```python
from build123d import *

# Parameters (mm, degrees)
CROQUIS1_W              = 53
CROQUIS1_H              = 24
CROQUIS1_R              = 8.15
CROQUIS1_W_2            = 10.3
CROQUIS1_H_2            = 4
CROQUIS1_W_3            = 9
CROQUIS1_H_3            = 2.5
SALIENTE_EXTRUIR1_DEPTH = 2
CROQUIS2_W              = 53
CROQUIS2_H              = 2
SALIENTE_EXTRUIR2_DEPTH = 16
SALIENTE_EXTRUIR3_DEPTH = 2
SALIENTE_EXTRUIR5_START = -53
SALIENTE_EXTRUIR5_DEPTH = 2
CROQUIS5_R              = 1.65
CROQUIS5_R_2            = 2
CORTAR_EXTRUIR1_DEPTH   = 2
REDONDEO1_R             = 2
REDONDEO6_R             = 1


with BuildPart() as part:
    # Croquis1 → Saliente-Extruir1 (new body)
    with BuildSketch(Plane.XY):
        with Locations((26.5, 12)):
            Rectangle(CROQUIS1_W, CROQUIS1_H)
        with Locations((13.5, 12)):
            Circle(CROQUIS1_R, mode=Mode.SUBTRACT)
        with Locations((39.5, 12)):
            Circle(CROQUIS1_R, mode=Mode.SUBTRACT)
        with Locations((26.5, 19)):
            Rectangle(CROQUIS1_W_2, CROQUIS1_H_2, mode=Mode.SUBTRACT)
        with Locations((26.5, 3.25)):
            Rectangle(CROQUIS1_W_3, CROQUIS1_H_3, mode=Mode.SUBTRACT)
    extrude(amount=SALIENTE_EXTRUIR1_DEPTH)

    # Croquis2 → Saliente-Extruir2 (add)
    with BuildSketch(Plane.XY.offset(2)):
        with Locations((26.5, -1)):
            Rectangle(CROQUIS2_W, CROQUIS2_H)
    extrude(amount=-SALIENTE_EXTRUIR2_DEPTH)

    # Croquis4 → Saliente-Extruir3 (add)
    with BuildSketch(Plane(origin=(53, 0, 0), x_dir=(0, 0, -1), z_dir=(1, 0, 0))):
        Polygon((14, -2), (14, 0), (0, 24), (-2, 24), (-2, -2), align=None)
    extrude(amount=-SALIENTE_EXTRUIR3_DEPTH)

    # Croquis4<3> → Saliente-Extruir5 (add)
    with BuildSketch(Plane(origin=(53, 0, 0), x_dir=(0, 0, -1), z_dir=(1, 0, 0)).offset(SALIENTE_EXTRUIR5_START)):
        Polygon((14, -2), (14, 0), (0, 24), (-2, 24), (-2, -2), align=None)
    extrude(amount=SALIENTE_EXTRUIR5_DEPTH)

    # Croquis5 → Cortar-Extruir1 (cut)
    with BuildSketch(Plane(origin=(0, 0, 0), x_dir=(1, 0, 0), z_dir=(0, 1, 0))):
        with Locations(Location((12.9, 10, 0), (0, 0, 270))):
            Circle(CROQUIS5_R)
        with Locations(Location((40.1, 10, 0), (0, 0, 270))):
            Circle(CROQUIS5_R)
        with Locations(Location((26.5, 10, 0), (0, 0, 270))):
            Circle(CROQUIS5_R_2)
    extrude(amount=-CORTAR_EXTRUIR1_DEPTH, mode=Mode.SUBTRACT)

    # Redondeo1
    redondeo1_edges = [part.edges().sort_by_distance(p)[0] for p in [
        (0, 24, 1),
        (53, 24, 1),
    ]]
    fillet(redondeo1_edges, radius=REDONDEO1_R)

    # Redondeo6
    redondeo6_edges = [part.edges().sort_by_distance(p)[0] for p in [
        (53, 10, 2),
        (0, 10, 2),
        (26.5, 24, 2),
        (52.414213562, 23.414213562, 2),
        (0.585786438, 23.414213562, 2),
    ]]
    fillet(redondeo6_edges, radius=REDONDEO6_R)


solid = part.part
```
The model under review builds one solid part; all positions refer to its coordinate system, in mm. A direction names the side the tool comes from. Give positions to 0.01 mm unless a question says otherwise; leave off trailing zeros. Loops run counter-clockwise (first coordinate to the right, second up) from the corner with the lowest first, then second, coordinate; pieces in that order, holes last. Notation, with made-up numbers: (28.25, 86) -> (42.25, 86) arc R26 ccw to (42.25, 123) -> close; hole circle Ø10 at (18, -18.5). An arc over 180 degrees is marked (long way). Use CSV: the item, a comma, the result in double quotes.
1. Consider section A-A, the plane x = 30. Write out the cut boundary in (y, z).
Result:
outline,"(-2, -14) -> (0, -14) -> (0, 0) -> (2, 0) -> (2, 2) -> (-2, 2) -> close; (4.5, 0) -> (17, 0) -> (17, 2) -> (4.5, 2) -> close; (21, 0) -> (24, 0) -> (24, 1) arc R1 ccw to (23, 2) -> (21, 2) -> close"
2. Consider section B-B, the plane z = -9. Write out the cut boundary in (x, y), then the cut area to 3 significant figures.
Result:
outline,"(0, -2) -> (11.59, -2) -> (11.59, 0) -> (2, 0) -> (2, 8.57) -> (0, 8.57) -> close; (14.21, -2) -> (24.77, -2) -> (24.77, 0) -> (14.21, 0) -> close; (28.23, -2) -> (38.79, -2) -> (38.79, 0) -> (28.23, 0) -> close; (41.41, -2) -> (53, -2) -> (53, 8.57) -> (51, 8.57) -> (51, 0) -> (41.41, 0) -> close"
area,"123 mm²"
3. Consider section C-C, the plane y = 11. Write out the cut boundary in (x, z).
Result:
outline,"(0, -7.58) -> (2, -7.58) -> (2, 0) -> (5.41, 0) -> (5.41, 2) -> (1, 2) arc R1 ccw to (0, 1) -> close; (21.59, 0) -> (31.41, 0) -> (31.41, 2) -> (21.59, 2) -> close; (47.59, 0) -> (51, 0) -> (51, -7.58) -> (53, -7.58) -> (53, 1) arc R1 ccw to (52, 2) -> (47.59, 2) -> close"
4. The part is to be moulded in two halves that separate along Z. For faces 1 (the face through (26, 11, 2)), 2 (the face through (14.29, -0.99, -9.11)), 3 (the face through (26, 12, 0)), 4 (the face through (26, 4.5, 1)), say which applies: +Z half, -Z half, draft (parallel to the pull), parting line (faces both ways), or undercut.
Result:
face 1,"+Z half"
face 2,"undercut"
face 3,"-Z half"
face 4,"draft"
5. To check wall thickness, follow probe 1 along X at (y, z) = (-1.25, -10); probe 2 along X at (y, z) = (2.25, -3.25); probe 3 along Z at (x, y) = (41, 21.75). State the ranges of each line that lie inside material, in increasing order. Write a range as from..to.
Result:
probe 1,"x = 0..11.25, 14.55..24.5, 28.5..38.45, 41.75..53"
probe 2,"x = 0..2, 51..53"
probe 3,"z = 0..2"
6. Machinability: for faces 5 (the face through (22, 3, 1)), 6 (the face through (26.2, 24, 0.5)), 7 (the face through (2, 7, -4)), which of the approach directions +Z, -Z, +X, -X, +Y, -Y give a long, thin tool a straight path to every point of the face, cutting with its end or side? Answer none if there is none.
Result:
face 5,"+Z, -Z"
face 6,"+Z, -Z, +X, -X, +Y"
face 7,"-Z, +Y"
7. Consider section D-D, the plane x = 18. Write out the cut boundary in (y, z), then the cut area to 3 significant figures.
Result:
outline,"(-2, -14) -> (0, -14) -> (0, 0) -> (5.2, 0) -> (5.2, 2) -> (-2, 2) -> close; (18.8, 0) -> (24, 0) -> (24, 1) arc R1 ccw to (23, 2) -> (18.8, 2) -> close"
area,"52.6 mm²"
8. For P1, Ø10, axis at x = 12.5, y = 19.5, coming from the -Z side; P2, Ø7, axis at x = 24, z = -4, coming from the +Y side, all flat-tipped, find the tip position at first contact; note any pin that passes through.
Result:
P1,"stops at z = 0"
P2,"stops at y = 0"
